Verification items for the finished model (mm, model axes). Give positions to 0.01 mm unless a question says otherwise; leave off trailing zeros. Loops run counter-clockwise (first coordinate to the right, second up) from the corner with the lowest first, then second, coordinate; pieces in that order, holes last. Notation, with made-up numbers: M 2,-34.5 L 35,-34.5 A27 ccw 35,-1.5 Z; hole C 2.25,68 d1. An arc over 180 degrees is marked long. Use a Markdown table: item, result.
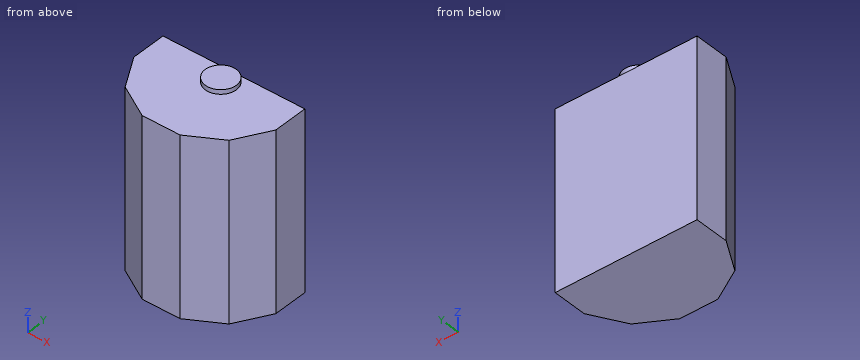
from build123d import *

# Parameters (mm, degrees)
F1_DEPTH = 254
F2_R     = 22.225
F3_DEPTH = 6.35


with BuildPart() as f1:
    # F0 (on Top) → F1 (new body)
    with BuildSketch(Plane.XY):
        Polygon((101.6, -27.223638), (101.6, 22.225), (0, 22.225), (-101.6, 22.225), (-101.6, -27.223638), (-74.376362, -74.376362), (-27.223638, -101.6), (27.223638, -101.6), (74.376362, -74.376362), align=None)
    extrude(amount=F1_DEPTH)

    # F2 (on face) → F3 (join)
    with BuildSketch(Plane.XY.offset(254)):
        Circle(F2_R)
    extrude(amount=F3_DEPTH)


solid = f1.part
(1) Cross-section at C-C on x = -39. Record the cut outline in (y, z) (3 decimals), then the cut area to 3 significant figures.
Results below:
| item | result |
|---|---|
| outline | M -94.801,0 L 22.225,0 L 22.225,254 L -94.801,254 Z |
| area | 29,700 mm^2 |
(2) Gauge pin test, flat ends, axial feed: P1, Ø10, axis at x = -35, y = -1, coming from the +Z side; P2, Ø2, axis at y = -56.5, z = 136.5, coming from the +X side; P3, Ø12, axis at y = -61.5, z = 95, coming from the -X side. Record the tip position at first contact, or that the pin passes through.
Results below:
| item | result |
|---|---|
| P1 | z = 254 |
| P2 | x = 85.27 |
| P3 | x = -85.27 |
(3) Material ranges on line 1 (Z direction, x = -30, y = 13.5); line 2 (Y direction, x = -92, z = 30.5) (3 decimals); line 3 (X direction, y = -71, z = 223.5), recorded low to high.
Results below:
| item | result |
|---|---|
| line 1 | 0 to 254 |
| line 2 | -43.851 to 22.225 |
| line 3 | -76.33 to 76.33 |
(4) Cross-section at B-B on y = 0. Record the cut outline in (x, z) (3 decimals), then the cut area to 3 significant figures.
Results below:
| item | result |
|---|---|
| outline | M -101.6,0 L 101.6,0 L 101.6,254 L 22.225,254 L 22.225,260.35 L -22.225,260.35 L -22.225,254 L -101.6,254 Z |
| area | 51,900 mm^2 |
(5) Cross-section at A-A on z = 54. Record the cut outline in (x, y) (3 decimals), then the cut area to 3 significant figures.
Results below:
| item | result |
|---|---|
| outline | M -101.6,-27.224 L -74.376,-74.376 L -27.224,-101.6 L 27.224,-101.6 L 74.376,-74.376 L 101.6,-27.224 L 101.6,22.225 L -101.6,22.225 Z |
| area | 21,100 mm^2 |
(6) Cross-section at D-D on y = -50. Record the cut outline in (x, z), then the cut area to 3 significant figures.
Results below:
| item | result |
|---|---|
| outline | M -88.45,0 L 88.45,0 L 88.45,254 L -88.45,254 Z |
| area | 44,900 mm^2 |
